Read the model definition and answer for the solid it produces. Units are mm, in the model's axes. A direction names the side the tool comes from. Coordinates: 2 decimals unless noted, no trailing zeros. Loops run counter-clockwise (first coordinate to the right, second up) from the corner with the lowest first, then second, coordinate; pieces in that order, holes last.
from build123d import *

# Parameters (mm, degrees)
SKETCH_W        = 450.8
SKETCH_H        = 64
PAD_DEPTH       = 15
SKETCH001_W     = 30
SKETCH001_H     = 64
POCKET_DEPTH    = 7.5
POCKET001_DEPTH = 3.75
POCKET002_DEPTH = 15.001
SKETCH005_R     = 1.5
POCKET004_DEPTH = 15.001
SKETCH006_W     = 410.8
SKETCH006_H     = 4
POCKET005_DEPTH = 7.5
SKETCH007_R     = 1.5
POCKET006_DEPTH = 15.001
POCKET007_DEPTH = 7.5
SKETCH010_R     = 3
POCKET009_DEPTH = 3


with BuildPart() as part:
    # Sketch → Pad (new body)
    with BuildSketch(Plane.XZ):
        with Locations((205.4, 32)):
            Rectangle(SKETCH_W, SKETCH_H)
    extrude(amount=PAD_DEPTH)

    # Sketch001 (on DatumPlane) → Pocket (cut)
    with BuildSketch(Plane.XZ):
        with Locations((15, 32)):
            Rectangle(SKETCH001_W, SKETCH001_H)
        with Locations((395.8, 32)):
            Rectangle(SKETCH001_W, SKETCH001_H)
    extrude(amount=POCKET_DEPTH, mode=Mode.SUBTRACT)

    # Sketch002 (on DatumPlane) → Pocket001 (cut)
    with BuildSketch(Plane.XZ.offset(15)):
        with BuildLine():
            Line((279.8, 55.5), (279.8, 8.5))
            ThreePointArc((279.8, 8.5), (280.092893, 7.792893), (280.8, 7.5))
            Line((280.8, 7.5), (378.8, 7.5))
            ThreePointArc((378.8, 7.5), (379.507107, 7.792893), (379.8, 8.5))
            Line((379.8, 8.5), (379.8, 35.500007))
            ThreePointArc((380.8, 36.500007), (380.092893, 36.207114), (379.8, 35.500007))
            Line((380.8, 36.500007), (409.8, 36.500007))
            ThreePointArc((409.8, 36.500007), (410.507102, 36.792895), (410.8, 37.499993))
            Line((410.8, 37.499993), (410.8, 44))
            Line((410.8, 44), (410.8, 50.500007))
            ThreePointArc((410.8, 50.500007), (410.507107, 51.207114), (409.8, 51.500007))
            Line((409.8, 51.500007), (380.8, 51.500007))
            ThreePointArc((379.8, 52.500007), (380.092893, 51.7929), (380.8, 51.500007))
            Line((379.8, 55.5), (379.8, 52.500007))
            ThreePointArc((379.8, 55.5), (379.507107, 56.207107), (378.8, 56.5))
            Line((378.8, 56.5), (280.8, 56.5))
            ThreePointArc((280.8, 56.5), (280.092893, 56.207107), (279.8, 55.5))
        make_face()
    extrude(amount=-POCKET001_DEPTH, mode=Mode.SUBTRACT)

    # Sketch003 (on DatumPlane) → Pocket002 (cut, through all)
    with BuildSketch(Plane.XZ.offset(15)):
        with BuildLine():
            Line((381.8, 51.5), (409.8, 51.5))
            ThreePointArc((410.8, 50.5), (410.507107, 51.207107), (409.8, 51.5))
            Line((410.8, 50.5), (410.8, 37.5))
            ThreePointArc((409.8, 36.5), (410.507107, 36.792893), (410.8, 37.5))
            Line((409.8, 36.5), (381.8, 36.5))
            ThreePointArc((380.8, 37.5), (381.092893, 36.792893), (381.8, 36.5))
            Line((380.8, 37.5), (380.8, 44))
            Line((380.8, 44), (380.8, 50.5))
            ThreePointArc((381.8, 51.5), (381.092893, 51.207107), (380.8, 50.5))
        make_face()
    extrude(amount=-POCKET002_DEPTH, mode=Mode.SUBTRACT)

    # Sketch005 (on DatumPlane) → Pocket004 (cut, through all)
    with BuildSketch(Plane.XZ.offset(15)):
        with Locations((287.3, 49)):
            Circle(SKETCH005_R)
        with Locations((287.3, 15)):
            Circle(SKETCH005_R)
        with Locations((372.3, 49)):
            Circle(SKETCH005_R)
        with Locations((372.3, 15)):
            Circle(SKETCH005_R)
    extrude(amount=-POCKET004_DEPTH, mode=Mode.SUBTRACT)

    # Sketch006 (on DatumPlane) → Pocket005 (cut)
    with BuildSketch(Plane.XZ):
        with Locations((205.4, 22)):
            Rectangle(SKETCH006_W, SKETCH006_H)
    extrude(amount=POCKET005_DEPTH, mode=Mode.SUBTRACT)

    # Sketch007 (on DatumPlane) → Pocket006 (cut, through all)
    with BuildSketch(Plane.XZ):
        with Locations((7.5, 56.5)):
            Circle(SKETCH007_R)
        with Locations((7.5, 31.5)):
            Circle(SKETCH007_R)
        with Locations((7.5, 10)):
            Circle(SKETCH007_R)
        with Locations((22.5, 56.5)):
            Circle(SKETCH007_R)
        with Locations((22.5, 31.5)):
            Circle(SKETCH007_R)
        with Locations((22.5, 10)):
            Circle(SKETCH007_R)
        with Locations((388.3, 56.5)):
            Circle(SKETCH007_R)
        with Locations((388.3, 31.5)):
            Circle(SKETCH007_R)
        with Locations((388.3, 10)):
            Circle(SKETCH007_R)
        with Locations((403.3, 56.5)):
            Circle(SKETCH007_R)
        with Locations((403.3, 31.5)):
            Circle(SKETCH007_R)
        with Locations((403.3, 10)):
            Circle(SKETCH007_R)
        with Locations((-10, 56.5)):
            Circle(SKETCH007_R)
        with Locations((-10, 31.5)):
            Circle(SKETCH007_R)
        with Locations((-10, 10)):
            Circle(SKETCH007_R)
        with Locations((420.8, 56.5)):
            Circle(SKETCH007_R)
        with Locations((420.8, 31.5)):
            Circle(SKETCH007_R)
        with Locations((420.8, 10)):
            Circle(SKETCH007_R)
    extrude(amount=POCKET006_DEPTH, mode=Mode.SUBTRACT)

    # Sketch008 (on DatumPlane) → Pocket007 (cut)
    with BuildSketch(Plane.XZ.offset(15)):
        with BuildLine():
            Line((378.8, 56.5), (280.8, 56.5))
            ThreePointArc((280.8, 56.5), (280.092893, 56.207107), (279.8, 55.5))
            Line((279.8, 55.5), (279.8, 52.5))
            ThreePointArc((278.8, 51.5), (279.507107, 51.792893), (279.8, 52.5))
            Line((278.8, 51.5), (1, 51.5))
            ThreePointArc((1, 51.5), (0.292893, 51.207107), (0, 50.5))
            Line((0, 50.5), (0, 37.5))
            ThreePointArc((0, 37.5), (0.292893, 36.792893), (1, 36.5))
            Line((1, 36.5), (278.8, 36.5))
            ThreePointArc((279.8, 35.5), (279.507107, 36.207107), (278.8, 36.5))
            Line((279.8, 35.5), (279.8, 28))
            ThreePointArc((279.8, 28), (280.092893, 27.292893), (280.8, 27))
            Line((280.8, 27), (378.8, 27))
            ThreePointArc((378.8, 27), (379.507107, 27.292893), (379.8, 28))
            Line((379.8, 35.5), (379.8, 28))
            ThreePointArc((380.8, 36.5), (380.092893, 36.207107), (379.8, 35.5))
            Line((380.8, 36.5), (409.8, 36.5))
            ThreePointArc((409.8, 36.5), (410.507107, 36.792893), (410.8, 37.5))
            Line((410.8, 37.5), (410.8, 44))
            Line((410.8, 44), (410.8, 50.5))
            ThreePointArc((410.8, 50.5), (410.507107, 51.207107), (409.8, 51.5))
            Line((409.8, 51.5), (380.8, 51.5))
            ThreePointArc((379.8, 52.5), (380.092893, 51.792893), (380.8, 51.5))
            Line((379.8, 55.5), (379.8, 52.5))
            ThreePointArc((379.8, 55.5), (379.507107, 56.207107), (378.8, 56.5))
        make_face()
    extrude(amount=-POCKET007_DEPTH, mode=Mode.SUBTRACT)

    # Sketch010 (on DatumPlane) → Pocket009 (cut)
    with BuildSketch(Plane.XZ):
        with Locations((287.3, 49)):
            Circle(SKETCH010_R)
        with Locations((372.3, 49)):
            Circle(SKETCH010_R)
        with Locations((287.3, 15)):
            Circle(SKETCH010_R)
        with Locations((372.3, 15)):
            Circle(SKETCH010_R)
    extrude(amount=POCKET009_DEPTH, mode=Mode.SUBTRACT)


solid = part.part
Item 1: Given pin 1 (5 mm diameter, centred on x = -10, z = 31.5, fed in from -Y); pin 2 (2.5 mm diameter, centred on x = 388.3, z = 10, fed in from +Y); pin 3 (5 mm diameter, centred on x = 372.3, z = 15, fed in from +Y); pin 4 (5 mm diameter, centred on x = 7.5, z = 31.5, fed in from +Y), each flat-ended and moving along its own axis, determine where each tip first touches the part or whether it passes through.
Numbers:
pin 1: stops at y = -15
pin 2: passes through
pin 3: stops at y = -3
pin 4: stops at y = -7.5
Item 2: A cutting plane is placed at A-A on x = 109. Determine the outline of the cut face in (y, z), then the cut area to 4 significant figures.
Numbers:
outline: (-15, 0) - (0, 0) - (0, 20) - (-7.5, 20) - (-7.5, 24) - (0, 24) - (0, 64) - (-15, 64) - (-15, 51.5) - (-7.5, 51.5) - (-7.5, 36.5) - (-15, 36.5) - close
area: 817.5 mm2
Item 3: Determine the mould class of faces 6 (the face through (203, -4, 20)), 7 (the face through (138, -11, 36.5)), 8 (the face through (202, -7, 0)), 9 (the face through (152, -15, 32)) for opening direction Z: released by +Z, released by -Z, zero draft, split by the parting line, or undercut.
Numbers:
face 6: undercut
face 7: undercut
face 8: released by -Z
face 9: zero draft
Item 4: Which of the six approach directions +Z, -Z, +X, -X, +Y, -Y give full straight-line access (tool end or side, diameter ignored) to faces 1 (the face through (410.8, -6, 32)), 2 (the face through (279.8, -12, 25)), 3 (the face through (395, -11, 36.5)), 4 (the face through (423, 0, 32)), 5 (the face through (380.8, -4, 44))?
Numbers:
face 1: +Y
face 2: -Y
face 3: +Y, -Y
face 4: +Z, -Z, +X, -X, +Y
face 5: +Z, -Z, +Y
Item 5: Find the intervals of material crossed by line 1 along X through (y, z) = (-1.5, 25); line 2 along Z through (x, y) = (287.3, -1.65); line 3 along Z through (x, y) = (287.3, -5.5), in increasing order.
Numbers:
line 1: x = -20 to 0, 30 to 380.8, 410.8 to 430.8
line 2: z = 0 to 12, 18 to 20, 24 to 46, 52 to 64
line 3: z = 0 to 13.5, 16.5 to 20, 24 to 47.5, 50.5 to 64
